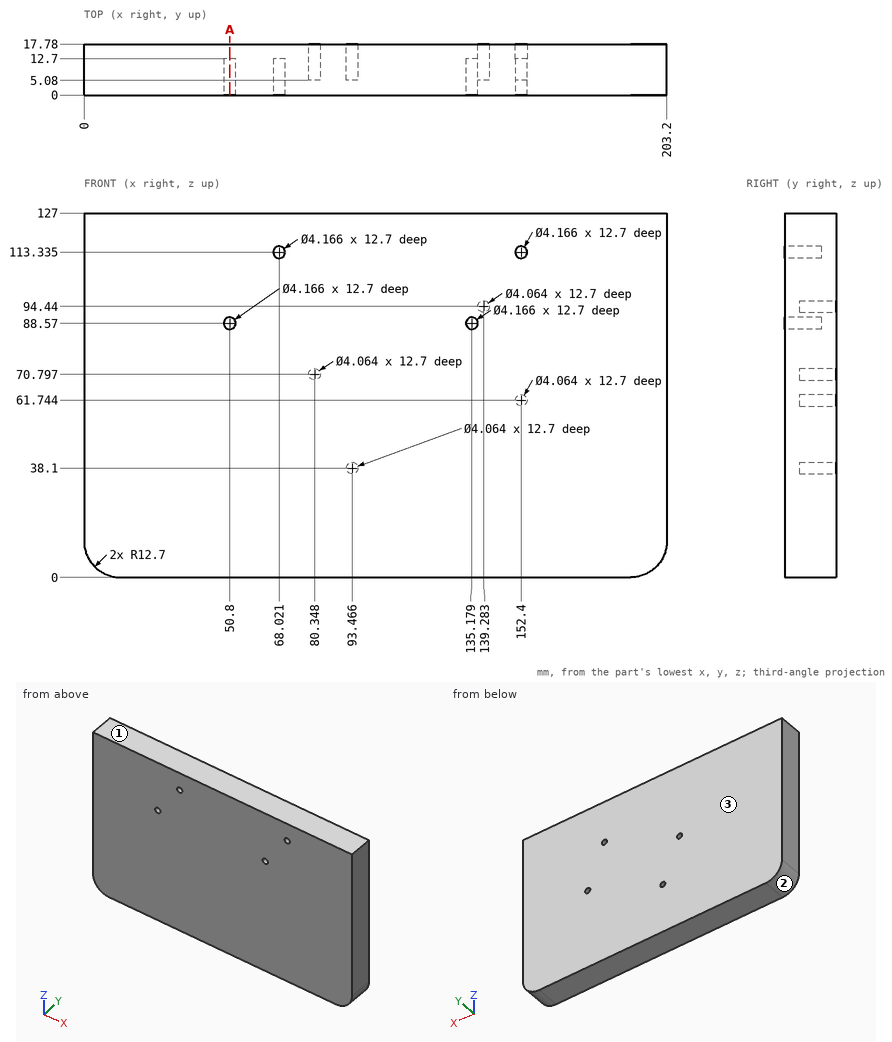
Print and shaded views of the part. All mm, measured from the part's lowest x, y and z. Round coordinates to 2 decimals unless told otherwise and drop trailing zeros. Write each loop counter-clockwise with the first axis right and the second up, starting at its lowest first coordinate (ties: lowest second). Pieces come first, ordered by that corner, then holes.
Item 1: Two-plate mould, pull along Z, no slides. Class the marked faces 1, 2 and 3: +Z half, -Z half, draft (parallel to the pull), parting line (faces both ways), or undercut.
Results:
face 1: +Z half
face 2: -Z half
face 3: draft
Item 2: Cut at A-A, the plane x = 50.8. Give the cut face in (y, z), plus the area to 4 significant figures.
Results:
outline: (0, 0) - (17.78, 0) - (17.78, 127) - (0, 127) - (0, 90.65) - (12.7, 90.65) - (12.7, 86.49) - (0, 86.49) - close
area: 2,205 mm2
Item 3: Drop flat-ended pins along their axis: pin 1 Ø3.5 at (x, z) = (139.28, 94.44) entering from +Y; pin 2 Ø1.2 at (x, z) = (135, 88) entering from -Y. Give the stop position or say it passes through.
Results:
pin 1: stops at y = 5.08
pin 2: stops at y = 12.7
Item 4: Probe L1, parallel to Z at x = 152.5, y = 9.5 (1 decimal); L2, parallel to X at y = 10.75, z = 62 (1 decimal); L3, parallel to X at y = 8.25, z = 38.1. List the from-to ranges inside material, lowest first.
Results:
L1: z = 0 to 59.7, 63.8 to 111.3, 115.4 to 127
L2: x = 0 to 150.4, 154.4 to 203.2
L3: x = 0 to 91.43, 95.5 to 203.2
